Autodesk Inventor part; units mm, degrees
ref_plane "YZ Plane" through (0, 0, 0) normal (1, 0, 0) x (0, 1, 0)
ref_plane "XZ Plane" through (0, 0, 0) normal (0, 1, 0) x (-1, 0, 0)
ref_plane "XY Plane" through (0, 0, 0) normal (0, 0, 1) x (1, 0, 0)
sketch "Sketch1" plane through (0, 0, 0) normal (1, 0, 0) x (0, 1, 0)
  line L0 (6.3049, 39.363) -> (-19.0951, 39.363)
  line L1 (-19.0951, 39.363) -> (-19.0951, -63.507)
  line L2 (-19.0951, -63.507) -> (6.3049, -63.507)
  line L3 (6.3049, -63.507) -> (6.3049, 39.363)
  point P0 (0, 0)
  dimension "d0" = 102.87
  dimension "d1" = 25.4
extrude "Extrusion1" add sketch "Sketch1" along normal blind 5.08
fillet "Fillet1" radius 6.35 2 edges at (2.54, 6.3049, 39.363) (2.54, 6.3049, -63.507)
sketch "Sketch7" plane through (0, -19.0951, 39.363) normal (0, 0, 1) x (1, 0, 0)
  line L0 (0, 0) -> (5.08, 0)
  line L1 (5.08, 0) -> (5.08, -5.08)
  line L2 (5.08, -5.08) -> (-33.02, -5.08)
  line L3 (-33.02, -5.08) -> (-33.02, 0)
  line L4 (-33.02, 0) -> (0, 0)
  line L5 (0, 0) -> (0, 0)
  line L6 (0, 0) -> (5.08, 0)
  line L7 (0, 19.05) -> (0, 0)
  point P0 (0, 19.0951)
  dimension "d51" = 5.08
  dimension "d52" = 5.08
  dimension "d53" = 90
  dimension "d54" = 5.08
  dimension "d55" = 38.1
  dimension "d56" = 0
  dimension "d57" = 0
extrude "Extrusion4" add sketch "Sketch7" against normal blind 102.87
fillet "Fillet2" radius 6.35 2 edges at (-33.02, -21.6351, -63.507) (-33.02, -21.6351, 39.363)
sketch "Sketch15" plane through (5.08, 0, 0) normal (1, 0, 0) x (0, 0, -1)
  line L0 (-39.363, -0.0451) -> (-39.363, -24.1751)
  line L1 (63.507, -0.0451) -> (63.507, -24.1751)
  line L2 (57.157, 6.3049) -> (-33.013, 6.3049)
  point P0 (0, 0)
  point P1 (-10.788, -6.3951)
  point P2 (34.2208, -6.3951)
  dimension "d143" = 0
  dimension "d144" = 45.0088
  dimension "d145" = 28.575
  dimension "d146" = 29.2862
  dimension "d147" = 12.7
hole "Hole7" at (5.08, -6.3951, 10.788) at (5.08, -6.3951, -34.2208) direction (-1, 0, 0) diameter 3.4036 depth 25.4 tip angle 118
sketch "Sketch16" plane through (5.08, -24.1751, -63.507) normal (0, -1, 0) x (1, 0, 0)
  line L0 (0, 102.87) -> (0, 0)
  line L1 (0, 102.87) -> (-31.75, 102.87)
  line L2 (-38.1, 96.52) -> (-38.1, 6.35)
  line L3 (0, 0) -> (-31.75, 0)
  point P0 (-5.08, 63.507)
  point P1 (-12.7, 96.52)
  point P2 (-31.75, 96.52)
  point P3 (-31.75, 6.35)
  point P4 (-12.7, 6.35)
  dimension "d155" = 0
  dimension "d156" = 0
  dimension "d157" = 0
  dimension "d158" = 0
  dimension "d159" = 12.7
  dimension "d160" = 6.35
  dimension "d161" = 6.35
  dimension "d162" = 6.35
hole "Hole8" at (-7.62, -24.1751, 33.013) at (-26.67, -24.1751, 33.013) at (-26.67, -24.1751, -57.157) at (-7.62, -24.1751, -57.157) direction (0, 1, 0) diameter 5.1054 depth 25.4 tip angle 118
properties part number "Realsense"
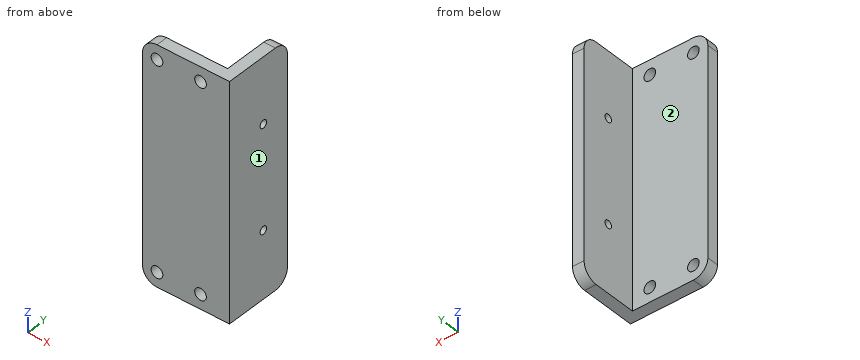
For this review, take the finished solid that the model builds, in its own axes (mm). Face numbers are marked on the shaded views. A direction names the side the tool comes from. Round coordinates to 2 decimals unless told otherwise and drop trailing zeros. Loops run counter-clockwise (first coordinate to the right, second up) from the corner with the lowest first, then second, coordinate; pieces in that order, holes last. Notation, with made-up numbers: (50, -17.75) - (59, -17.75) arc R29 ccw to (59, 4.25) - close; hole circle Ø8 at (24.25, -33.5). An arc over 180 degrees is marked (long way). Use one line per item in the form item = value.
Item 1: Clearance check with flat-ended pins moving along their axes: P1, Ø12, axis at x = -10.5, y = 0.5, coming from the -Z side; P2, Ø6.5, axis at x = -7.62, z = -57.157, coming from the +Y side; P3, Ø12.5, axis at y = -9.5, z = 6.5, coming from the -X side; P4, Ø10, axis at x = -25.5, y = -15.5, coming from the -Z side. State where each tip first meets the part, or that it passes through.
Answers:
P1 = through
P2 = -19.1
P3 = 0
P4 = -63.51
Item 2: For line 1 (Z direction, x = -7.62, y = -21.7); line 2 (Z direction, x = 3, y = -6); line 3 (X direction, y = 1.5, z = 7.5), list the stretches that pass through material, from the lowest coordinate up.
Answers:
line_1 = -63.51 to -59.71, -54.6 to 30.46, 35.57 to 39.36
line_2 = -63.51 to -35.88, -32.57 to 9.13, 12.44 to 39.36
line_3 = 0 to 5.08
Item 3: Consider section B-B on x = -7.62. Write out the cut boundary in (y, z), then the cut area to 3 significant figures.
Answers:
outline = (-24.18, -63.51) - (-19.1, -63.51) - (-19.1, -59.71) - (-24.18, -59.71) - close; (-24.18, -54.6) - (-19.1, -54.6) - (-19.1, 30.46) - (-24.18, 30.46) - close; (-24.18, 35.57) - (-19.1, 35.57) - (-19.1, 39.36) - (-24.18, 39.36) - close
area = 471 mm^2
Item 4: Tool access review of the marked faces 1 and 2: name each direction out of +Z, -Z, +X, -X, +Y, -Y from which nothing blocks a thin tool from reaching the whole face with its end or side.
Answers:
face_1 = +Z, -Z, +X, +Y, -Y
face_2 = +Z, -Z, -X, +Y
Item 5: Consider section D-D on y = -17.5. Write out the cut boundary in (x, z), then the cut area to 3 significant figures.
Answers:
outline = (0, -63.51) - (5.08, -63.51) - (5.08, 39.36) - (0, 39.36) - close
area = 523 mm^2
Item 6: Consider section C-C on z = 1.5. Write out the cut boundary in (x, y), then the cut area to 3 significant figures.
Answers:
outline = (-33.02, -24.18) - (5.08, -24.18) - (5.08, 6.3) - (0, 6.3) - (0, -19.1) - (-33.02, -19.1) - close
area = 323 mm^2
Item 7: Consider section A-A on y = -21.5. Write out the cut boundary in (x, z).
Answers:
outline = (-33.02, -57.16) arc R6.35 ccw to (-26.67, -63.51) - (5.08, -63.51) - (5.08, 39.36) - (-26.67, 39.36) arc R6.35 ccw to (-33.02, 33.01) - close; hole circle Ø5.11 at (-26.67, -57.16); hole circle Ø5.11 at (-26.67, 33.01); hole circle Ø5.11 at (-7.62, -57.16); hole circle Ø5.11 at (-7.62, 33.01)
